```python
from build123d import *

# Parameters (mm, degrees)
F0_W           = 50
F0_H           = 3
F1_DEPTH       = 150
F3_START       = 51
F2_R           = 6
F2_R_2         = 3
F3_DEPTH       = 48
F5_D           = 5
F5_CSINK_D     = 10
F5_CSINK_ANGLE = 90


# Not quite as in the source:
# - a feature names something its author has since deleted; it is built from what else it names


with BuildPart() as f1:
    # F0 (on Top) → F1 (new body)
    with BuildSketch(Plane.XY):
        with Locations((25, 1.5)):
            Rectangle(F0_W, F0_H)
    extrude(amount=F1_DEPTH)

    # F2 (on Top) → F3 (join)
    with BuildSketch(Plane.XY.offset(F3_START)):
        with Locations((-5.8086630434, 1.5)):
            Circle(F2_R)
        with Locations((-5.8086630434, 1.5)):
            Circle(F2_R_2, mode=Mode.SUBTRACT)
    extrude(amount=F3_DEPTH)

    # F5 (through all)
    with Locations(Plane.XZ):
        with Locations((38.6542826891, 135), (15, 75), (38.6542826891, 15)):
            CounterSinkHole(F5_D / 2, F5_CSINK_D / 2, counter_sink_angle=F5_CSINK_ANGLE)


solid = f1.part
```
Model file for the job. Use its own axes, mm. A direction names the side the tool comes from. Coordinates: 2 decimals unless noted, no trailing zeros. Loops run counter-clockwise (first coordinate to the right, second up) from the corner with the lowest first, then second, coordinate; pieces in that order, holes last. Notation, with made-up numbers: (57, -22.5) -> (71, -22.5) arc R18 cw to (71, 8.5) -> close; hole circle Ø6 at (85.25, 73). An arc over 180 degrees is marked (long way). Answer as a JSON object with one key per item and string values.
Q1. Cut at B-B (z = 15). List the corners of the cut face in (x, y), and give its area (3 significant figures).
Report:
{"outline": "(0, 0) -> (33.65, 0) -> (36.15, 2.5) -> (36.15, 3) -> (0, 3) -> close; (41.15, 2.5) -> (43.65, 0) -> (50, 0) -> (50, 3) -> (41.15, 3) -> close", "area": "129 mm2"}
Q2. Cut at A-A (x = 15). List the corners of the cut face in (y, z).
Report:
{"outline": "(0, 0) -> (3, 0) -> (3, 72.5) -> (2.5, 72.5) -> (0, 70) -> close; (0, 80) -> (2.5, 77.5) -> (3, 77.5) -> (3, 150) -> (0, 150) -> close"}
Q3. Cut at C-C (z = 56.5). List the corners of the cut face in (x, y).
Report:
{"outline": "(0, 0) -> (50, 0) -> (50, 3) -> (0, 3) arc R6 ccw (long way) to start; hole circle Ø6 at (-5.81, 1.5)"}
Q4. Pull direction Z, two halves, no side cores. Call faces 4 (the cylindrical face through (-11.804, 1.743, 74.664)), 5 (the conical face through (41.27, 2.38, 15.12)), 6 (the flat face through (25, 2, 150)): released by +Z, released by -Z, zero draft, split by the parting line, or undercut.
Report:
{"face 4": "zero draft", "face 5": "undercut", "face 6": "released by +Z"}
Q5. Probe probe 1 along X at (y, z) = (2.85, 135); probe 2 along X at (y, z) = (2.6, 75); probe 3 along Y at (x, z) = (-6, 65). List the from-to ranges inside material, lowest first.
Report:
{"probe 1": "x = 0 to 36.15, 41.15 to 50", "probe 2": "x = -11.71 to -8.6, -3.02 to 12.5, 17.5 to 50", "probe 3": "y = -4.5 to -1.49, 4.49 to 7.5"}
Q6. Flat gauge pins, fed straight in: P1, Ø1, axis at y = 6, z = 82.5, coming from the -X side; P2, Ø15, axis at x = 36.5, z = 65, coming from the +Y side; P3, Ø2.5, axis at y = 1, z = 135, coming from the -X side; P4, Ø4.5, axis at x = 38.65, z = 15, coming from the -Y side. Where does each tip first touch, or does it go through?
Report:
{"P1": "stops at x = -10.28", "P2": "stops at y = 3", "P3": "stops at x = 0", "P4": "passes through"}
Q7. Cut at D-D (x = 25.5). List the corners of the cut face in (y, z), and give its area (3 significant figures).
Report:
{"outline": "(0, 0) -> (3, 0) -> (3, 150) -> (0, 150) -> close", "area": "450 mm2"}
Q8. 3-axis set-ups, long thin cutter, end or side, ignore diameter. For faces 1 (the flat face through (25, 0, 74)), 2 (the flat face through (-9, 0, 99)), 3 (the flat face through (25, 3, 74)): which of +Z, -Z, +X, -X, +Y, -Y reach the whole face in a straight line?
Report:
{"face 1": "+Z, -Z, +X, -Y", "face 2": "+Z, -X, +Y, -Y", "face 3": "+Z, -Z, +X, +Y"}
